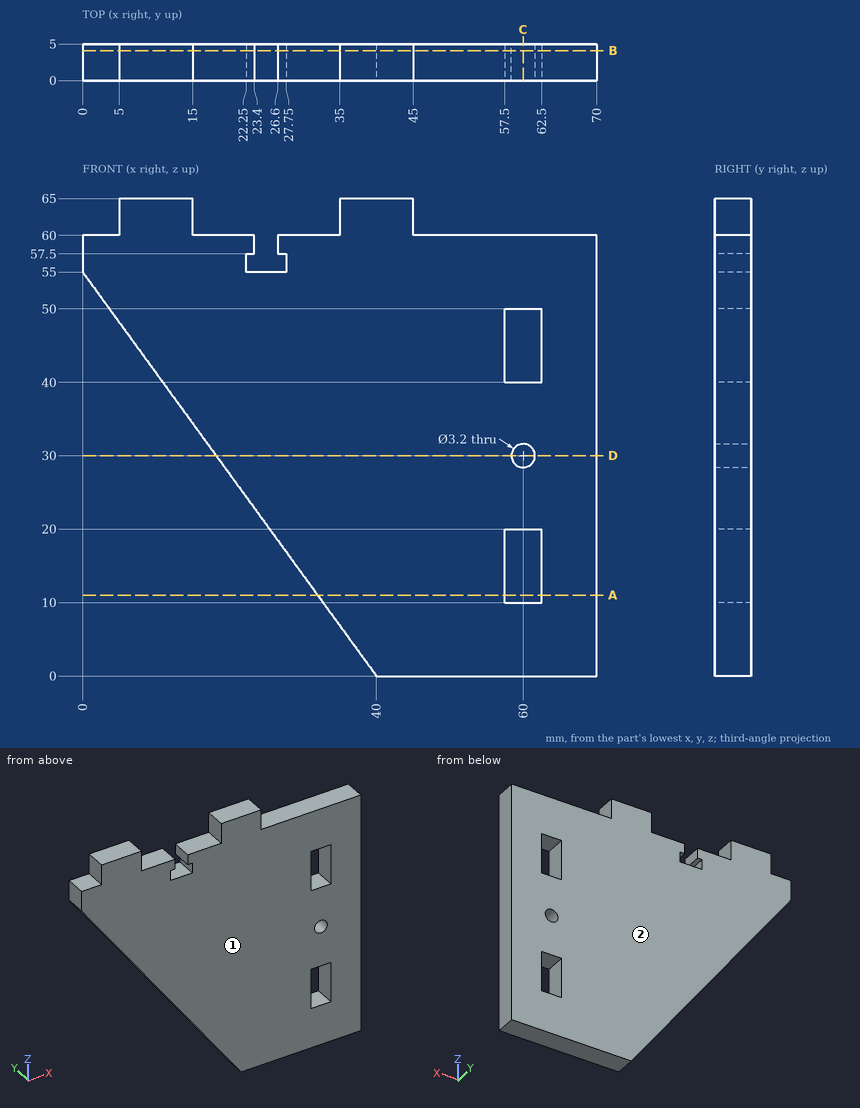
Can you work these out from the drawing? Everything is in mm from the part's minimum corner. Coordinates: 2 decimals unless noted, no trailing zeros. Loops run counter-clockwise (first coordinate to the right, second up) from the corner with the lowest first, then second, coordinate; pieces in that order, holes last. Notation, with made-up numbers: (3, 61.25) - (44, 61.25) arc R19 ccw to (44, 78.25) - close; hole circle Ø8 at (68.5, 1.5). An arc over 180 degrees is marked (long way). Use a Markdown table: item, result.
Item 1: If I drill on probe 1 along Z at (x, y) = (60, 1.7); probe 2 along Z at (x, y) = (59, 0.5); probe 3 along X at (y, z) = (2.8, 48), over which ranges is the centre line in solid material (lowest first)? Write a range as from..to.
Numbers:
| item | result |
|---|---|
| probe 1 | z = 0..10, 20..28.4, 31.6..40, 50..60 |
| probe 2 | z = 0..10, 20..28.75, 31.25..40, 50..60 |
| probe 3 | x = 5.09..57.5, 62.5..70 |
Item 2: We'd pull the mould along Y, two halves only. Please class the marked faces 1 and 2: released by +Y, released by -Y, zero draft, split by the parting line, or undercut.
Numbers:
| item | result |
|---|---|
| face 1 | released by -Y |
| face 2 | released by +Y |
Item 3: I want a section at B-B on y = 4.1. Give the number of separate pieces and of enclosed holes in the cut face, and give its area (3 significant figures).
Numbers:
| item | result |
|---|---|
| separate pieces | 1 |
| enclosed holes | 3 |
| area | 3,070 mm2 |
Item 4: I want a section at D-D on z = 30. Please give me the cut outline in (x, y).
Numbers:
| item | result |
|---|---|
| outline | (18.18, 0) - (58.4, 0) - (58.4, 5) - (18.18, 5) - close; (61.6, 0) - (70, 0) - (70, 5) - (61.6, 5) - close |
Item 5: Will these pins go through, and if not, where does the flat tip stop? pin 1 (2.5 mm diameter, centred on x = 21, y = 2, fed in from +Z); pin 2 (0.9 mm diameter, centred on x = 27.5, y = 2.5, fed in from -Z); pin 3 (1.5 mm diameter, centred on y = 1.5, z = 46.5, fed in from -X).
Numbers:
| item | result |
|---|---|
| pin 1 | stops at z = 60 |
| pin 2 | stops at z = 16.57 |
| pin 3 | stops at x = 5.64 |
Item 6: I want a section at C-C on x = 60. Please give me the cut outline in (y, z), and give its area (3 significant figures).
Numbers:
| item | result |
|---|---|
| outline | (0, 0) - (5, 0) - (5, 10) - (0, 10) - close; (0, 20) - (5, 20) - (5, 28.4) - (0, 28.4) - close; (0, 31.6) - (5, 31.6) - (5, 40) - (0, 40) - close; (0, 50) - (5, 50) - (5, 60) - (0, 60) - close |
| area | 184 mm2 |
Item 7: I want a section at A-A on z = 11. Please give me the cut outline in (x, y), and give its area (3 significant figures).
Numbers:
| item | result |
|---|---|
| outline | (32, 0) - (57.5, 0) - (57.5, 5) - (32, 5) - close; (62.5, 0) - (70, 0) - (70, 5) - (62.5, 5) - close |
| area | 165 mm2 |
